```python
from build123d import *

# Parameters (mm, degrees)
SKETCH1_R                  = 20
BOSS_EXTRUDE1_DEPTH        = 40
SKETCH3_R                  = 4
CUT_EXTRUDE1_DEPTH         = 30
M4X0_7_TAPPED_HOLE1_REACH  = 50.99
M4X0_7_TAPPED_HOLE1_BORE_R = 1.65
SKETCH4_W                  = 5
SKETCH4_H                  = 5
CUT_EXTRUDE2_DEPTH         = 0.5


with BuildPart() as part:
    # Sketch1 → Boss-Extrude1 (new body)
    with BuildSketch(Plane(origin=(0, 0, 0), x_dir=(1, 0, 0), z_dir=(0, 1, 0))):
        with Locations(Location((0, 0, 0), (0, 0, 270))):
            Circle(SKETCH1_R)
    extrude(amount=BOSS_EXTRUDE1_DEPTH)

    # Sketch3 → Cut-Extrude1 (cut)
    with BuildSketch(Plane(origin=(0, 0, -20), x_dir=(-1, 0, 0), z_dir=(0, 0, -1))):
        with Locations((0, 20)):
            Circle(SKETCH3_R)
    extrude(amount=-CUT_EXTRUDE1_DEPTH, mode=Mode.SUBTRACT)

    # M4x0.7 Tapped Hole1 bore (on position points) → M4x0.7 Tapped Hole1 (cut, up to next)
    with BuildSketch(Plane(origin=(20, 20, 0), x_dir=(0, 0, 1), z_dir=(1, 0, 0)), mode=Mode.PRIVATE) as m4x0_7_tapped_hole1_sk1:
        Circle(M4X0_7_TAPPED_HOLE1_BORE_R)
    m4x0_7_tapped_hole1_tool1 = extrude(m4x0_7_tapped_hole1_sk1.sketch, amount=-M4X0_7_TAPPED_HOLE1_REACH, mode=Mode.PRIVATE) & part.part
    add(m4x0_7_tapped_hole1_tool1.solids().sort_by_distance((20, 20, 0))[0], mode=Mode.SUBTRACT)

    # Sketch4 → Cut-Extrude2 (cut)
    with BuildSketch(Plane(origin=(20, 0, 0), x_dir=(0, 0, -1), z_dir=(1, 0, 0))):
        with Locations((0, 20)):
            Rectangle(SKETCH4_W, SKETCH4_H)
    extrude(amount=-CUT_EXTRUDE2_DEPTH, mode=Mode.SUBTRACT)


solid = part.part
```
Could you check a few things on this model? Use its own coordinates, in mm. A direction names the side the tool comes from. Coordinates: 2 decimals unless noted, no trailing zeros. Loops run counter-clockwise (first coordinate to the right, second up) from the corner with the lowest first, then second, coordinate; pieces in that order, holes last.
1) Imagine slicing it at A-A (z = 0). List the corners of the cut face in (x, y) for me, and give its area (3 significant figures).
Reported:
outline: (-20, 0) - (20, 0) - (20, 17.5) - (19.5, 17.5) - (19.5, 18.35) - (3.64, 18.35) arc R4 cw (long way) to (3.64, 21.65) - (19.5, 21.65) - (19.5, 22.5) - (20, 22.5) - (20, 40) - (-20, 40) - close
area: 1,500 mm2
2) Thinking about a two-plate mould opening in Y: for faces 4 (the face through (0, 40, 0)), 5 (the face through (0, 0, 0)), 6 (the face through (0, 20, 10)), which applies, released by +Y, released by -Y, zero draft, split by the parting line, or undercut?
Reported:
face 4: released by +Y
face 5: released by -Y
face 6: undercut
3) Which directions (+Z, -Z, +X, -X, +Y, -Y) give clear straight access to the entire face, cutting with the end or side of a thin tool? Please do faces 1 (the face through (19.5, 22, 0)), 2 (the face through (6.007, 19.72, 19.076)), 3 (the face through (-3.815, 21.201, -5.21)).
Reported:
face 1: +X
face 2: +Y, -Y
face 3: -Z
4) Please list where these lines run through material, in increasing order: line 1 along Y through (x, z) = (0, -12); line 2 along Z through (x, y) = (16, 20); line 3 along X through (y, z) = (22.5, -16.5).
Reported:
line 1: y = 0 to 16, 24 to 40
line 2: z = -12 to -1.65, 1.65 to 12
line 3: x = -11.3 to -3.12, 3.12 to 11.3
5) Will these pins go through, and if not, where does the flat tip stop? pin 1 Ø5 at (y, z) = (18.5, 11.5) entering from -X; pin 2 Ø6.5 at (x, y) = (-0.5, 20.5) entering from -Z; pin 3 Ø8 at (y, z) = (27.5, 3.5) entering from -X.
Reported:
pin 1: stops at x = -17.86
pin 2: stops at z = 10
pin 3: stops at x = -20
6) Imagine slicing it at B-B (y = 20). List the corners of the cut face in (x, z) for me, and give its area (3 significant figures).
Reported:
outline: (-4, -19.6) - (-4, 10) - (4, 10) - (4, 1.65) - (19.5, 1.65) - (19.5, 2.5) - (19.84, 2.5) arc R20 ccw (long way) to start; (4, -19.6) arc R20 ccw to (19.84, -2.5) - (19.5, -2.5) - (19.5, -1.65) - (4, -1.65) - close
area: 964 mm2
7) Imagine slicing it at C-C (x = 0). List the corners of the cut face in (y, z) for me, and give its area (3 significant figures).
Reported:
outline: (0, -20) - (16, -20) - (16, 10) - (24, 10) - (24, -20) - (40, -20) - (40, 20) - (0, 20) - close
area: 1,360 mm2
8) Imagine slicing it at D-D (x = 15). List the corners of the cut face in (y, z) for me.
Reported:
outline: (0, -13.23) - (40, -13.23) - (40, 13.23) - (0, 13.23) - close; hole circle Ø3.3 at (20, 0)
